```python
from build123d import *

# Parameters (mm, degrees)
SKETCH1_R           = 7
SKETCH1_R_2         = 4
BOSS_EXTRUDE1_DEPTH = 8
CHAMFER1_SIZE       = 0.2
CHAMFER2_SIZE       = 2
CHAMFER2_SIZE2      = 1.154700538


with BuildPart() as part:
    # Sketch1 → Boss-Extrude1 (new body)
    with BuildSketch(Plane.XY):
        Circle(SKETCH1_R)
        Circle(SKETCH1_R_2, mode=Mode.SUBTRACT)
    extrude(amount=BOSS_EXTRUDE1_DEPTH)

    # Chamfer1
    chamfer1_edges = [part.edges().sort_by_distance(p)[0] for p in [
        (-7, 0, 8),
    ]]
    chamfer(chamfer1_edges, length=CHAMFER1_SIZE)

    # Chamfer2
    chamfer2_edges = [part.edges().sort_by_distance(p)[0] for p in [
        (-7, 0, 0),
    ]]
    chamfer2_side = [part.faces().sort_by_distance(p)[0] for p in [
        (-6.802010101, 0, 0),
    ]]
    chamfer(chamfer2_edges, length=CHAMFER2_SIZE, length2=CHAMFER2_SIZE2, reference=chamfer2_side[0])


solid = part.part
```
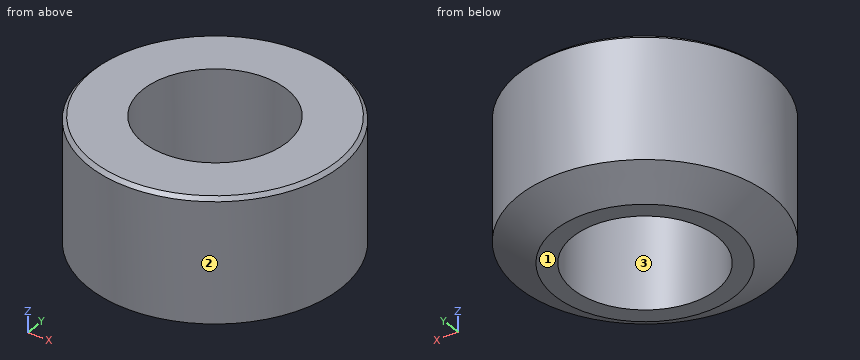
Geometry check sheet. Reference: the model listing, model coordinates, mm. Face numbers are marked on the shaded views. Coordinates: 2 decimals unless noted, no trailing zeros. Loops run counter-clockwise (first coordinate to the right, second up) from the corner with the lowest first, then second, coordinate; pieces in that order, holes last.
Item 1: Thickness scan on line 1 (Y direction, x = 0, z = 4.5); line 2 (X direction, y = -3, z = 7); line 3 (Y direction, x = -1.25, z = 6). Record the ranges inside material, lowest first.
Item 2: Release check for a two-part mould opening along X. For the marked faces 1, 2 and 3 record: released by +X, released by -X, zero draft, split by the parting line, or undercut.
Item 3: Sectioned sample at C-C, the plane z = 6.25. Record the boundary of the cut face in (x, y), then the cut area to 3 significant figures.
Item 4: Sectioned sample at A-A, the plane y = 0. Record the boundary of the cut face in (x, z), then the cut area to 3 significant figures.
Item 5: Go/stop test with flat-tipped pins: pin 1 Ø2 at (y, z) = (4.5, 6.5) entering from +X; pin 2 Ø2 at (x, z) = (-5.5, 5.5) entering from +Y. Record where each tip stops, or that it passes through.
Check result:
1. line 1: y = -7 to -4, 4 to 7
1. line 2: x = -6.32 to -2.65, 2.65 to 6.32
1. line 3: y = -6.89 to -3.8, 3.8 to 6.89
2. face 1: zero draft
2. face 2: split by the parting line
2. face 3: undercut
3. outline: circle Ø14 at (0, 0); hole circle Ø8 at (0, 0)
3. area: 104 mm2
4. outline: (-7, 1.15) - (-5, 0) - (-4, 0) - (-4, 8) - (-6.8, 8) - (-7, 7.8) - close; (4, 0) - (5, 0) - (7, 1.15) - (7, 7.8) - (6.8, 8) - (4, 8) - close
4. area: 45.7 mm2
5. pin 1: stops at x = 6.06
5. pin 2: stops at y = 5.36
